The model under review builds one solid part; all positions refer to its coordinate system, in mm. A direction names the side the tool comes from. Give positions to 0.01 mm unless a question says otherwise; leave off trailing zeros. Order: outer loops, then holes, each group sorted by start corner. A loop starts at its lowest first (then second) coordinate and runs counter-clockwise, first axis right, second up.
```python
from build123d import *

# Parameters (mm, degrees)
SKETCH_2_R          = 11
EXTRUDE_1_DEPTH     = 15
SKETCH_3_R          = 2.5
CUT_EXTRUDE_1_DEPTH = 34.793490497
SKETCH_4_R          = 5
CUT_EXTRUDE_2_DEPTH = 20


with BuildPart() as part:
    # 스케치2 → 보스-돌출1 (new, symmetric)
    with BuildSketch(Plane(origin=(0, 0, 0), x_dir=(1, 0, 0), z_dir=(0, 1, 0))):
        with Locations(Location((0, 0, 0), (0, 0, 270))):
            Circle(SKETCH_2_R)
    extrude(amount=EXTRUDE_1_DEPTH, both=True)

    # 스케치3 → 컷-돌출1 (cut, through all)
    with BuildSketch(Plane.XZ.offset(15)):
        with Locations(Location((0, 0, 0), (0, 0, 270))):
            Circle(SKETCH_3_R)
    extrude(amount=-CUT_EXTRUDE_1_DEPTH, mode=Mode.SUBTRACT)

    # 스케치4 → 컷-돌출2 (cut)
    with BuildSketch(Plane(origin=(0, 15, 0), x_dir=(1, 0, 0), z_dir=(0, 1, 0))):
        with Locations(Location((0, 0, 0), (0, 0, 270))):
            Circle(SKETCH_4_R)
    extrude(amount=-CUT_EXTRUDE_2_DEPTH, mode=Mode.SUBTRACT)


solid = part.part
```
Item 1: Take a section at A-A (z = 0). Give the boundary of the cut face in (x, y).
Values found:
outline: (-11, -15) - (-2.5, -15) - (-2.5, -5) - (-5, -5) - (-5, 15) - (-11, 15) - close; (2.5, -15) - (11, -15) - (11, 15) - (5, 15) - (5, -5) - (2.5, -5) - close
Item 2: Draft analysis for pull direction X (two halves, no side actions). For faces 1 (the flat face through (-5, 15, 2)), 2 (the cylindrical face through (-2.44, -10.07, 0.54)), 3 (the cylindrical face through (-10.74, 0.21, -2.38)), state which applies: released by +X, released by -X, zero draft, split by the parting line, or undercut.
Values found:
face 1: zero draft
face 2: undercut
face 3: split by the parting line
Item 3: Take a section at D-D (x = -4.25). Give the boundary of the cut face in (y, z).
Values found:
outline: (-15, -10.15) - (15, -10.15) - (15, -2.63) - (-5, -2.63) - (-5, 2.63) - (15, 2.63) - (15, 10.15) - (-15, 10.15) - close
Item 4: For line 1 (X direction, y = 1.25, z = 0); line 2 (X direction, y = -8.25, z = 0); line 3 (Z direction, x = 3.25, y = 4.75), list the stretches that pass through material, from the lowest coordinate up.
Values found:
line 1: x = -11 to -5, 5 to 11
line 2: x = -11 to -2.5, 2.5 to 11
line 3: z = -10.51 to -3.8, 3.8 to 10.51
Item 5: Take a section at C-C (y = -4.5). Give the boundary of the cut face in (x, z), and give its area (3 significant figures).
Values found:
outline: circle Ø22 at (0, 0); hole circle Ø10 at (0, 0)
area: 302 mm2
Item 6: Take a section at B-B (x = 0). Give the boundary of the cut face in (y, z).
Values found:
outline: (-15, -11) - (15, -11) - (15, -5) - (-5, -5) - (-5, -2.5) - (-15, -2.5) - close; (-15, 2.5) - (-5, 2.5) - (-5, 5) - (15, 5) - (15, 11) - (-15, 11) - close
Item 7: For faces 4 (the flat face through (0, -15, -3)), 5 (the flat face through (-2, -5, 2)), list the 3-axis set-ups (+Z, -Z, +X, -X, +Y, -Y) from which the entire face can be reached by the end or side of a thin tool; tool diameter is ignored.
Values found:
face 4: +Z, -Z, +X, -X, -Y
face 5: +Y
Item 8: Clearance check with flat-ended pins moving along their axes: pin 1 Ø4 at (x, y) = (5, -11) entering from +Z; pin 2 Ø8 at (x, z) = (0, 0) entering from -Y; pin 3 Ø1 at (y, z) = (0, -5.5) entering from -X; pin 4 Ø1 at (x, y) = (-6, -1) entering from +Z. State where each tip first meets the part, or that it passes through.
Values found:
pin 1: stops at z = 10.58
pin 2: stops at y = -15
pin 3: stops at x = -9.8
pin 4: stops at z = 9.53
